Autodesk Inventor part; units mm, degrees
ref_plane "YZ Plane" through (0, 0, 0) normal (1, 0, 0) x (0, 1, 0)
ref_plane "XZ Plane" through (0, 0, 0) normal (0, 1, 0) x (-1, 0, 0)
ref_plane "XY Plane" through (0, 0, 0) normal (0, 0, 1) x (1, 0, 0)
sketch "Sketch1" plane through (0, 0, 0) normal (0, 0, 1) x (1, 0, 0)
  line L0 (0, 0) -> (525.78, 0)
  line L1 (525.78, 0) -> (525.78, 101.6)
  line L2 (525.78, 101.6) -> (0, 101.6)
  line L3 (0, 101.6) -> (0, 0)
  line L4 (0, 101.6) -> (262.89, 253.3796)
  line L5 (262.89, 253.3796) -> (525.78, 101.6)
  point P0 (262.89, 101.6)
  dimension "d0" = 525.78
  dimension "d1" = 101.6
  dimension "d2" = 30
extrude "Extrusion1" add sketch "Sketch1" along normal blind 6.35
sketch "Sketch7" plane through (0, 0, 6.35) normal (0, 0, 1) x (1, 0, 0)
  circle A0 centre (262.89, 121.3796) radius 60
  point P0 (0, 0)
  point P1 (262.89, 253.3796)
  dimension "d26" = 120
  dimension "d30" = 132
extrude "Extrusion7" cut sketch "Sketch7" against normal through all
properties part number "BA10" material "ABS Plastic"
For this review, take the finished solid that the model builds, in its own axes (mm). Coordinates: 2 decimals unless noted, no trailing zeros. Loops run counter-clockwise (first coordinate to the right, second up) from the corner with the lowest first, then second, coordinate; pieces in that order, holes last. Notation, with made-up numbers: (-21, -32) - (30, -32) arc R24 cw to (30, -3) - close; hole circle Ø3 at (88.5, -24.75). An arc over 180 degrees is marked (long way). Use one line per item in the form item = value. Start each with the question number.
1) Take a section at A-A (z = 2). State the section outline as (x, y) points.
2) Draft analysis for pull direction X (two halves, no side actions). For faces 1 (the face through (218.668, 161.93, 3.219)), 2 (the face through (259, 44, 0)), 3 (the face through (392.495, 178.552, 3.131)), state which applies: released by +X, released by -X, zero draft, split by the parting line, or undercut.
3) To check wall thickness, follow probe 1 along Y at (x, z) = (262.89, 4.5); probe 2 along Y at (x, z) = (223, 1.5); probe 3 along X at (y, z) = (98, 3.25). State the ranges of each line that lie inside material, in increasing order. Write a range as from..to.
4) Take a section at C-C (y = 221). State the section outline as (x, z) points, plus the area to 3 significant figures.
5) Take a section at B-B (x = 172). State the section outline as (y, z) points, plus the area to 3 significant figures.
6) For pin 1 (3 mm diameter, centred on y = 190, z = 4.5, fed in from +X), flat-tipped, find the tip position at first contact; note if it passes through.
From the geometry:
q1.outline = (0, 0) - (525.78, 0) - (525.78, 101.6) - (262.89, 253.38) - (0, 101.6) - close; hole circle Ø120 at (262.89, 121.38)
q2.face_1 = undercut
q2.face_2 = zero draft
q2.face_3 = released by +X
q3.probe_1 = 0..61.38, 181.38..253.38
q3.probe_2 = 0..76.56, 166.2..230.35
q3.probe_3 = 0..207.63, 318.15..525.78
q4.outline = (206.81, 0) - (318.97, 0) - (318.97, 6.35) - (206.81, 6.35) - close
q4.area = 712 mm2
q5.outline = (0, 0) - (200.9, 0) - (200.9, 6.35) - (0, 6.35) - close
q5.area = 1,280 mm2
q6.pin_1 = 375.26
